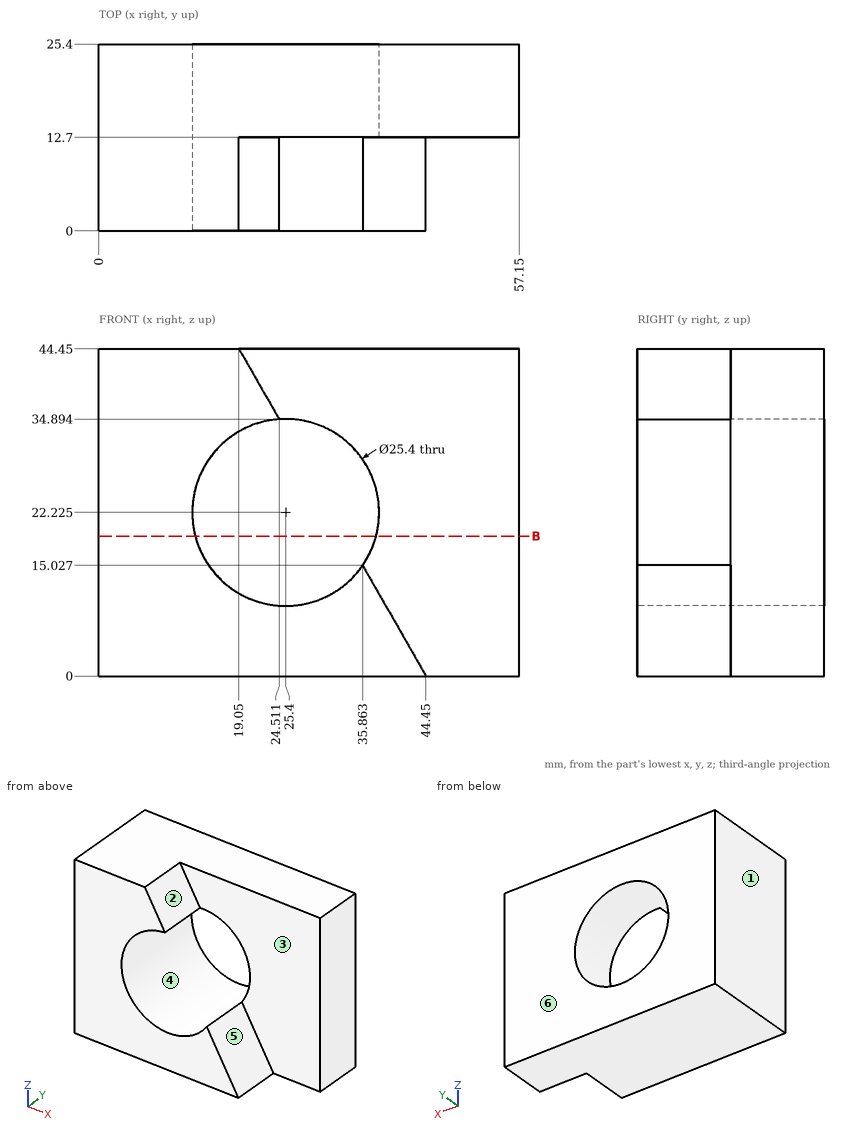
Job drawing, mm, ordinate dimensions from the low corner. One solid piece. A direction names the side the tool comes from. Coordinates: 2 decimals unless noted, no trailing zeros. Write each loop counter-clockwise with the first axis right and the second up, starting at its lowest first coordinate (ties: lowest second). Pieces come first, ordered by that corner, then holes.
Item 1: Slice it at B-B (z = 19). Write the cut outline in (x, y).
Item 2: Probe line 1 (X direction, y = 22.75, z = 31); line 2 (Y direction, x = 53.5, z = 6.5); line 3 (Z direction, x = 33, y = 18.5). List the from-to ranges inside material, lowest first.
Item 3: Which spindle directions (+Z, -Z, +X, -X, +Y, -Y) get a long thin tool onto all of the face, cutting with end or side? Do the marked faces 5 and 6. Say none if no direction does.
Item 4: Pin check, flat tips, straight feed: pin 1 (4 mm diameter, centred on x = 35, z = 29.5, fed in from +Y); pin 2 (10 mm diameter, centred on x = 46, z = 20.5, fed in from -Y). Stop position of each tip, or through.
Item 5: Mould opens along X. For the marked faces 1, 2, 3 and 4 say: released by +X, released by -X, zero draft, split by the parting line, or undercut.
Results found:
1. outline: (0, 0) - (13.12, 0) - (13.12, 25.4) - (0, 25.4) - close; (37.68, 12.7) - (57.15, 12.7) - (57.15, 25.4) - (37.68, 25.4) - close
2. line 1: x = 0 to 16.22, 34.58 to 57.15
2. line 2: y = 12.7 to 25.4
2. line 3: z = 0 to 12.05, 32.4 to 44.45
3. face 5: +Z, +X, -Y
3. face 6: +Z, -Z, +X, -X, +Y
4. pin 1: stops at y = 25.4
4. pin 2: stops at y = 12.7
5. face 1: released by -X
5. face 2: released by +X
5. face 3: zero draft
5. face 4: undercut
